Autodesk Inventor part; units mm, degrees
ref_plane "YZ Plane" through (0, 0, 0) normal (1, 0, 0) x (0, 1, 0)
ref_plane "XZ Plane" through (0, 0, 0) normal (0, 1, 0) x (-1, 0, 0)
ref_plane "XY Plane" through (0, 0, 0) normal (0, 0, 1) x (1, 0, 0)
sketch "Ecran" plane through (0, 0, 0) normal (0, 0, 1) x (1, 0, 0)
  line L0 (-38.59, 21.36) -> (38.59, 21.36)
  line L1 (38.59, 21.36) -> (38.59, 0)
  line L2 (-38.59, 0) -> (-38.59, 21.36)
  circle A0 centre (35.59, 18.36) radius 1.6
  line L3 (-38.59, 0) -> (38.59, 0)
  line L4 (35.59, 21.36) -> (35.59, 0)
  line L5 (-31.67, 21.36) -> (-31.67, 0)
  circle A1 centre (-31.67, 18.36) radius 1.6
  line L6 (-38.59, -21.36) -> (38.59, -21.36)
  line L7 (38.59, -21.36) -> (38.59, 0)
  line L8 (-38.59, 0) -> (-38.59, -21.36)
  circle A2 centre (35.59, -18.36) radius 1.6
  line L9 (35.59, -21.36) -> (35.59, 0)
  line L10 (-31.67, -21.36) -> (-31.67, 0)
  circle A3 centre (-31.67, -18.36) radius 1.6
  line L11 (32.08, 21.36) -> (-28.18, 21.36)
  line L12 (-28.18, 21.36) -> (-28.18, -21.36)
  line L13 (-28.18, -21.36) -> (32.08, -21.36)
  line L14 (32.08, -21.36) -> (32.08, 21.36)
  point P0 (0, 0)
  point P1 (38.59, 10.68)
  point P2 (35.59, 10.68)
  point P3 (38.59, -10.68)
  point P4 (35.59, -10.68)
  dimension "d3" = 3.2
  dimension "d4" = 3
  dimension "d5" = 77.18
  dimension "d6" = 21.36
  dimension "d8" = 67.26
  dimension "d9" = 3
  dimension "d12" = 60.26
  dimension "d13" = 6.51
extrude "Extrusion1" add sketch "Ecran" along normal blind 9 contours L0 L5 A1 L3 L2 | L0 L12 L3 L5 A1 | L3 L10 A3 L6 L8 | L0 L14 L3 L12 | L3 L12 L6 L10 A3 | L0 L4 A0 L3 L14 | L3 L14 L6 L12 | L0 L1 L3 L4 A0 | L3 L9 A2 L6 L14 | L3 L7 L6 L9 A2
sketch "Sketch3" plane through (0, 0, 9) normal (0, 0, 1) x (1, 0, 0)
  line L0 (38.59, 21.36) -> (-38.59, 21.36)
  line L1 (-38.59, -21.36) -> (38.59, -21.36)
  line L2 (38.59, 21.36) -> (32.08, 21.36)
  line L3 (32.08, 21.36) -> (32.08, -21.36)
  line L4 (32.08, -21.36) -> (38.59, -21.36)
  line L5 (38.59, -21.36) -> (38.59, 21.36)
  line L6 (32.08, -21.36) -> (-28.18, -21.36)
  line L7 (-28.18, -21.36) -> (-28.18, 21.36)
  line L8 (-28.18, 21.36) -> (32.08, 21.36)
  line L9 (32.08, 21.36) -> (32.08, -21.36)
  line L10 (-38.59, 21.36) -> (-38.59, -21.36)
  line L11 (-28.18, 21.36) -> (-38.59, 21.36)
  line L12 (-38.59, 21.36) -> (-38.59, -21.36)
  line L13 (-38.59, -21.36) -> (-28.18, -21.36)
  line L14 (-28.18, -21.36) -> (-28.18, 21.36)
  point P0 (0, 0)
  point P1 (38.59, -21.36)
  dimension "d14" = 6.51
  dimension "d15" = 60.26
extrude "Extrusion2" cut sketch "Sketch3" against normal blind 7 contours L5 L1 L3 L0 | L7 L1 L10 L0
properties part number "Ecran" material "Glass"
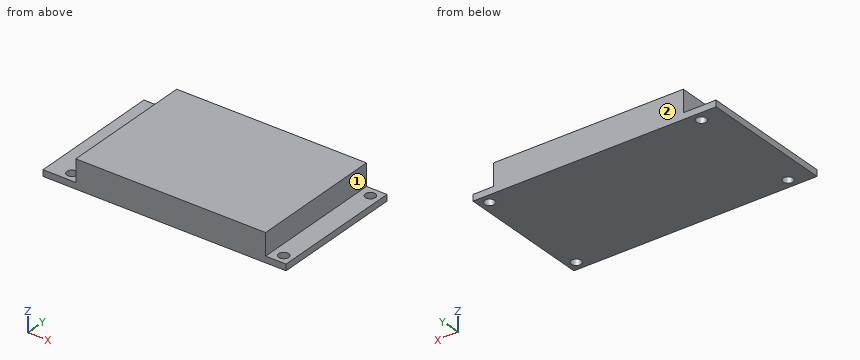
Part model, mm, in its own coordinate system. Face numbers are marked on the shaded views. A direction names the side the tool comes from. Give positions to 0.01 mm unless a question says otherwise; leave off trailing zeros. Loops run counter-clockwise (first coordinate to the right, second up) from the corner with the lowest first, then second, coordinate; pieces in that order, holes last. Notation, with made-up numbers: (-22.5, 88.5) -> (14.5, 88.5) arc R26 cw to (14.5, 123.5) -> close; hole circle Ø11 at (64.25, 38.25). An arc over 180 degrees is marked (long way). Write each question's results on one line, items separated by ' | '. Start each with the question number.
Q1. Band-saw the part on C-C on y = 2. List the corners of the cut face in (x, z), plus the area to 3 significant figures.
Q2. Band-saw the part on D-D on z = 8. List the corners of the cut face in (x, y), plus the area to 3 significant figures.
Q3. Pin check, flat tips, straight feed: P1, Ø3.5, axis at y = 0.5, z = 6.5, coming from the +X side; P2, Ø2, axis at y = -4, z = 7, coming from the -X side; P3, Ø5, axis at x = -31.67, y = -18.36, coming from the +Z side. Stop position of each tip, or through.
Q4. Wall check: L1, parallel to X at y = 18.36, z = 1.35; L2, parallel to Y at x = 35.59, z = 1.6; L3, parallel to X at y = -8, z = 3.25. Give the ranges that are in metal, low to high.
Q5. Band-saw the part on B-B on x = 35.59. List the corners of the cut face in (y, z), plus the area to 3 significant figures.
Q6. Which spindle directions (+Z, -Z, +X, -X, +Y, -Y) get a long thin tool onto all of the face, cutting with end or side? Do the marked faces 1 and 2. Say none if no direction does.
Q7. Band-saw the part on A-A on y = 18.36. List the corners of the cut face in (x, z).
Results are:
1) outline: (-38.59, 0) -> (38.59, 0) -> (38.59, 2) -> (32.08, 2) -> (32.08, 9) -> (-28.18, 9) -> (-28.18, 2) -> (-38.59, 2) -> close | area: 576 mm²
2) outline: (-28.18, -21.36) -> (32.08, -21.36) -> (32.08, 21.36) -> (-28.18, 21.36) -> close | area: 2,570 mm²
3) P1: stops at x = 32.08 | P2: stops at x = -28.18 | P3: stops at z = 2
4) L1: x = -38.59 to -33.27, -30.07 to 33.99, 37.19 to 38.59 | L2: y = -21.36 to -19.96, -16.76 to 16.76, 19.96 to 21.36 | L3: x = -28.18 to 32.08
5) outline: (-21.36, 0) -> (-19.96, 0) -> (-19.96, 2) -> (-21.36, 2) -> close; (-16.76, 0) -> (16.76, 0) -> (16.76, 2) -> (-16.76, 2) -> close; (19.96, 0) -> (21.36, 0) -> (21.36, 2) -> (19.96, 2) -> close | area: 72.6 mm²
6) face 1: +Z, +X, +Y, -Y | face 2: +Z, -Z, +X, -X, +Y
7) outline: (-38.59, 0) -> (-33.27, 0) -> (-33.27, 2) -> (-38.59, 2) -> close; (-30.07, 0) -> (33.99, 0) -> (33.99, 2) -> (32.08, 2) -> (32.08, 9) -> (-28.18, 9) -> (-28.18, 2) -> (-30.07, 2) -> close; (37.19, 0) -> (38.59, 0) -> (38.59, 2) -> (37.19, 2) -> close
